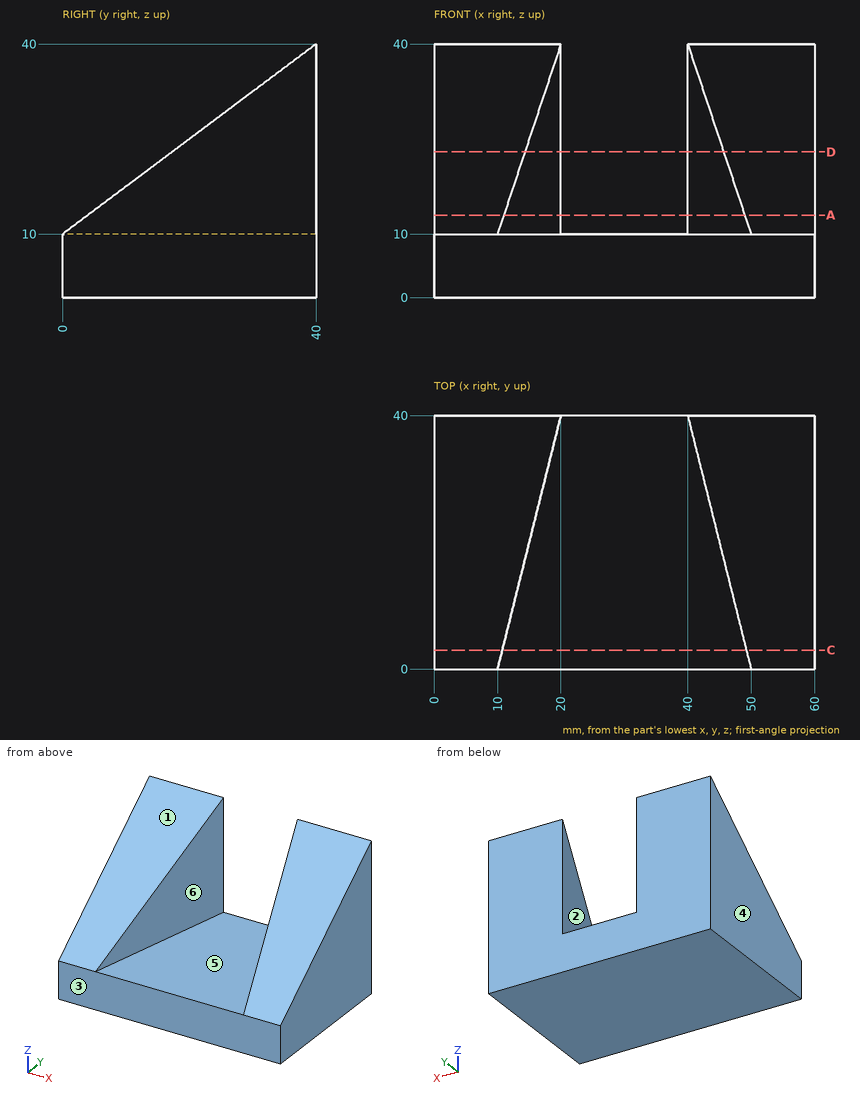
Could you check a few things on this drawing? It's one solid part, dimensions in mm from its lowest x, y, z. A direction names the side the tool comes from. Coordinates: 2 decimals unless noted, no trailing zeros. Order: outer loops, then holes, each group sorted by start corner. A loop starts at its lowest first (then second) coordinate and runs counter-clockwise, first axis right, second up. Notation, with made-up numbers: M 27.25,9.25 L 31.25,9.25 A16 ccw 31.25,14.25 Z; hole C 33.25,-19.5 d5. An arc over 180 degrees is marked long. Answer as a JSON object with one key per item and string values. Group by question number.
(1) For pin 1 (8 mm diameter, centred on x = 28, y = 7.5, fed in from +Z), with a flat end and sliding along its axis, tell me the tip position at first contact or that it passes through.
(2) If we mould it in two halves opening along X, with no side actions, what happens to the marked faces 3, 4, 5 and 6? For each: released by +X, released by -X, zero draft, split by the parting line, or undercut.
(3) Which directions (+Z, -Z, +X, -X, +Y, -Y) give clear straight access to the entire face, cutting with the end or side of a thin tool? Please do the marked faces 1 and 2.
(4) Suppose I cut it at D-D, the plane z = 23. Please give me the cut outline in (x, y).
(5) Suppose I cut it at A-A, the plane z = 13. Please give me the cut outline in (x, y).
(6) Suppose I cut it at C-C, the plane y = 3. Please give me the cut outline in (x, z).
(7) I need wall thicknesses on probe 1 along Z at (x, y) = (28.5, 13); probe 2 along X at (y, z) = (9, 12); probe 3 along X at (y, z) = (27.5, 14) (3 decimals). Which ranges of each line are inside material? Lowest first, please.
Values found:
{
 "1": {"pin 1": "stops at z = 10"},
 "2": {"face 3": "zero draft", "face 4": "released by -X", "face 5": "undercut", "face 6": "undercut"},
 "3": {"face 1": "+Z, +X, -X, -Y", "face 2": "+Z, -Y"},
 "4": {"outline": "M 0,17.33 L 14.33,17.33 L 20,40 L 0,40 Z; M 40,40 L 45.67,17.33 L 60,17.33 L 60,40 Z"},
 "5": {"outline": "M 0,4 L 11,4 L 20,40 L 0,40 Z; M 40,40 L 49,4 L 60,4 L 60,40 Z"},
 "6": {"outline": "M 0,0 L 60,0 L 60,12.25 L 49.25,12.25 L 49.25,10 L 10.75,10 L 10.75,12.25 L 0,12.25 Z"},
 "7": {"probe 1": "z = 0 to 10", "probe 2": "x = 0 to 12.25, 47.75 to 60", "probe 3": "x = 0 to 16.875, 43.125 to 60"}
}
